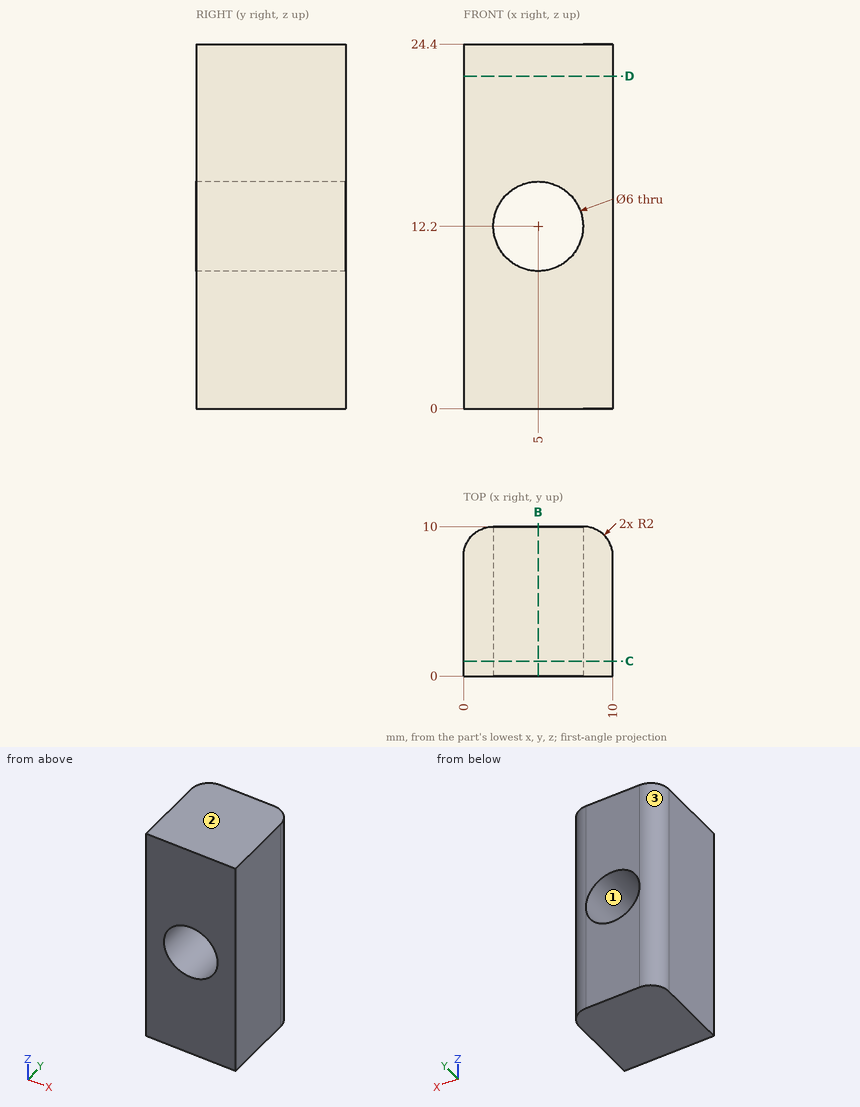
Source: three-view drawing plus pictorial views. Frame: mm from the lowest corner of the part. Round coordinates to 2 decimals unless told otherwise and drop trailing zeros. Write each loop counter-clockwise with the first axis right and the second up, starting at its lowest first coordinate (ties: lowest second). Pieces come first, ordered by that corner, then holes. Notation, with made-up numbers: M 23,-27.75 L 38,-27.75 A13 ccw 38,-2.75 Z; hole C 73.25,-2.75 d5. An arc over 180 degrees is marked long. Use CSV: the item, a comma, the result in double quotes. Start each with the question number.
Q1. Line query: line 1 (X direction, y = 5, z = 12.2); line 2 (X direction, y = 9.25, z = 14.5); line 3 (Z direction, x = 7, y = 1). Output: solid intervals per line, ascending. Write a range as from..to.
Q2. Pull-direction query (Z, two-part tool) for the marked faces 1, 2 and 3; classes: +Z half, -Z half, draft (parallel to the pull), parting line (faces both ways), or undercut.
Q3. Cut plane D-D on z = 22.25. Output: boundary loops of the cut face in (x, y).
Q4. Cut plane B-B on x = 5. Output: boundary loops of the cut face in (y, z).
Q5. Cut plane C-C on y = 1. Output: boundary loops of the cut face in (x, z), plus the area to 3 significant figures.
Results found:
1,line 1,"0..2, 8..10"
1,line 2,"0.44..3.07, 6.93..9.56"
1,line 3,"0..9.96, 14.44..24.4"
2,face 1,"undercut"
2,face 2,"+Z half"
2,face 3,"draft"
3,outline,"M 0,0 L 10,0 L 10,8 A2 ccw 8,10 L 2,10 A2 ccw 0,8 Z"
4,outline,"M 0,0 L 10,0 L 10,9.2 L 0,9.2 Z; M 0,15.2 L 10,15.2 L 10,24.4 L 0,24.4 Z"
5,outline,"M 0,0 L 10,0 L 10,24.4 L 0,24.4 Z; hole C 5,12.2 d6"
5,area,"216 mm^2"
